Verification items for this drawing (mm, ordinates from the low corner). A direction names the side the tool comes from. Round coordinates to 2 decimals unless told otherwise and drop trailing zeros. Loops run counter-clockwise (first coordinate to the right, second up) from the corner with the lowest first, then second, coordinate; pieces in that order, holes last. Notation, with made-up numbers: (65, 46.5) - (93, 46.5) arc R21 cw to (93, 78.5) - close; hole circle Ø5 at (47.5, 10.25). An arc over 180 degrees is marked (long way). Answer in a Markdown table with one row per item. Add a question column.
(1) Access from +Z, -Z, +X, -X, +Y, -Y to the whole of each face (thin tool, end or side, straight path). Record for the marked faces 4 and 5.
(2) Cross-section at A-A on y = 10. Enter the section's corners in (x, z).
(3) Mould release check, pull along X, two halves, no side actions. Record for the marked faces 1, 2 and 3: +X half, -X half, draft (parallel to the pull), parting line (faces both ways), or undercut.
(4) Cross-section at C-C on y = 5.25. Enter the section's corners in (x, z).
(5) Thickness scan on line 1 along Y through (x, z) = (10, 0.4); line 2 along X through (y, z) = (5, 1.9); line 3 along Y through (x, z) = (8.75, 0.3) (1 decimal). Record the ranges inside material, lowest first.
(6) Cross-section at D-D on x = 4.5. Enter the section's corners in (y, z).
(7) Gauge pin test, flat ends, axial feed: pin 1 (1 mm diameter, centred on x = 16.5, z = 1.5, fed in from -Y); pin 2 (0.6 mm diameter, centred on y = 4, z = 1, fed in from -X); pin 3 (2 mm diameter, centred on x = 14.5, z = 1, fed in from +Y). Record the tip position at first contact, or that the pin passes through.
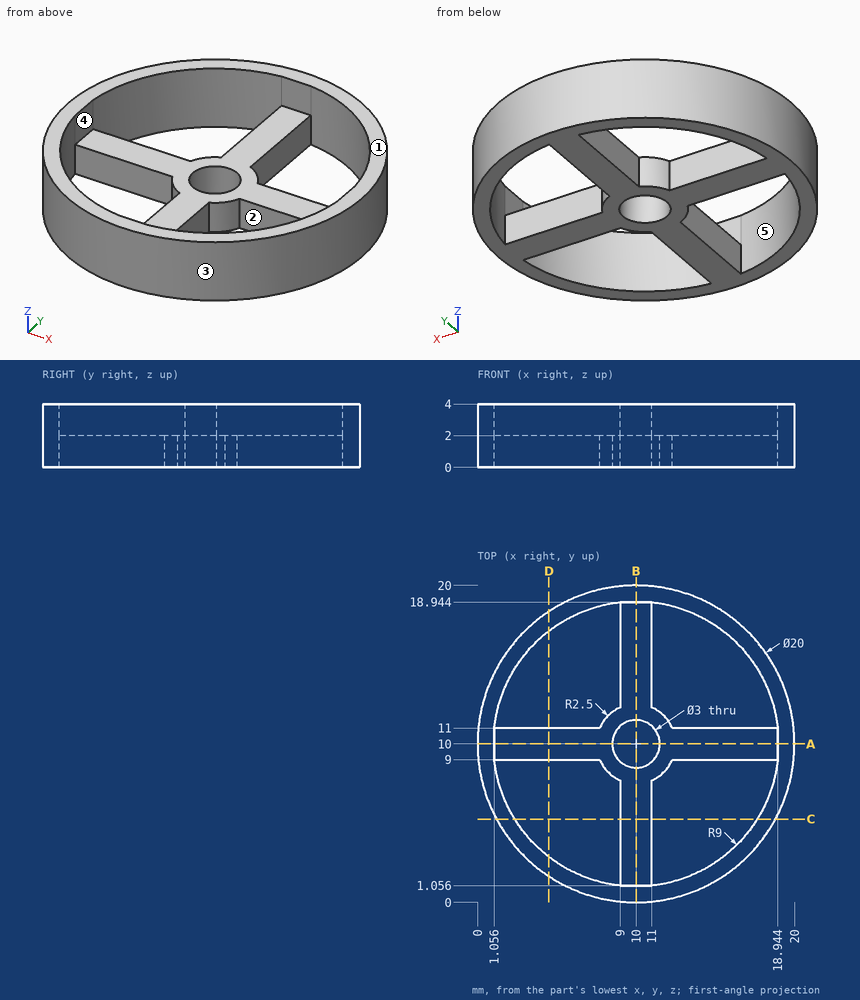
Answers:
| question | item | result |
|---|---|---|
| 1 | face 4 | +Z |
| 1 | face 5 | +Z, -Z |
| 2 | outline | (0, 0) - (8.5, 0) - (8.5, 2) - (1.06, 2) - (1.06, 4) - (0, 4) - close; (11.5, 0) - (20, 0) - (20, 4) - (18.94, 4) - (18.94, 2) - (11.5, 2) - close |
| 3 | face 1 | draft |
| 3 | face 2 | undercut |
| 3 | face 3 | parting line |
| 4 | outline | (1.2, 0) - (2.36, 0) - (2.36, 4) - (1.2, 4) - close; (9, 0) - (11, 0) - (11, 2) - (9, 2) - close; (17.64, 0) - (18.8, 0) - (18.8, 4) - (17.64, 4) - close |
| 5 | line 1 | y = 0 to 8.5, 11.5 to 20 |
| 5 | line 2 | x = 1.34 to 2.52, 9 to 11, 17.48 to 18.66 |
| 5 | line 3 | y = 0.1 to 1.1, 7.8 to 9.2, 10.8 to 12.2, 18.9 to 19.9 |
| 6 | outline | (1.65, 0) - (2.88, 0) - (2.88, 4) - (1.65, 4) - close; (9, 0) - (11, 0) - (11, 2) - (9, 2) - close; (17.12, 0) - (18.35, 0) - (18.35, 4) - (17.12, 4) - close |
| 7 | pin 1 | stops at y = 2 |
| 7 | pin 2 | stops at x = 1.78 |
| 7 | pin 3 | stops at y = 19.37 |
